Here's how the part is built. I have some questions about the finished solid (model axes, mm). Face numbers are marked on the shaded views. Round coordinates to 2 decimals unless told otherwise and drop trailing zeros. Loops run counter-clockwise (first coordinate to the right, second up) from the corner with the lowest first, then second, coordinate; pieces in that order, holes last. Notation, with made-up numbers: (-21, 0) - (21, 0) arc R16 ccw to (21, 16) - close; hole circle Ø10 at (31, 13). An arc over 180 degrees is marked (long way). Answer as a JSON object with one key per item and string values. Group by question number.
1) I want a section at C-C, the plane z = 1.55. Please give me the cut outline in (x, y).
2) I want a section at A-A, the plane y = 0. Please give me the cut outline in (x, z), then the cut area to 3 significant figures.
3) If I drill on line 1 along X through (y, z) = (0, 1.3); line 2 along Z through (x, y) = (5, 3); line 3 along X through (y, z) = (-8, 1.45), over which ranges is the centre line in solid material (lowest first)? Write a range as [from, to].
4) If we mould it in two halves opening along X, with no side actions, what happens to the marked faces 1 and 2? For each: pulls with the +X half, pulls with the -X half, needs draft (parallel to the pull), parting line crosses it, or undercut.
5) I want a section at B-B, the plane x = 0. Please give me the cut outline in (y, z), then the cut area to 3 significant figures.
6) Will these pins go through, and if not, where does the flat tip stop? P1, Ø8, axis at x = -4, y = 10, coming from the -Z side; P2, Ø1.5, axis at y = 15.5, z = 1.5, coming from the -X side; P3, Ø1.5, axis at x = -12, z = 1.5, coming from the +Y side; P4, Ø1, axis at x = -8, z = 2, coming from the +Y side.
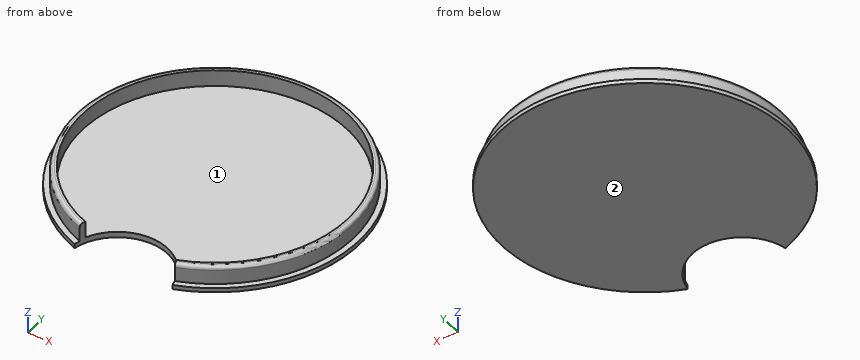
from build123d import *

# Parameters (mm, degrees)
F0_R     = 20
F1_DEPTH = 0.6
F3_R     = 19.2
F4_DEPTH = 2.5
F5_T     = -0.8
F6_R     = 0.5
F9_D     = 14
F9_DEPTH = 4


with BuildPart() as f1:
    # F0 (on Top) → F1 (new body)
    with BuildSketch(Plane.XY):
        Circle(F0_R)
    extrude(amount=F1_DEPTH)

    # F3 (on face) → F4 (join)
    with BuildSketch(Plane.XY.offset(0.6)):
        Circle(F3_R)
    extrude(amount=F4_DEPTH)

    # F5
    f5_openings = [f1.faces().sort_by_distance(p)[0] for p in [
        (0, 0, 3.1),
    ]]
    offset(amount=F5_T, openings=f5_openings)

    # F6
    f6_edges = [f1.edges().sort_by_distance(p)[0] for p in [
        (-19.2, 0, 3.1),
    ]]
    fillet(f6_edges, radius=F6_R)

    # F9
    with Locations(Plane.XY.offset(3.1)):
        with Locations((0, -20)):
            Hole(F9_D / 2, depth=F9_DEPTH)


solid = f1.part
Outcome:
{
 "1": {"outline": "(-6.71, -17.99) arc R7 cw to (-6.43, -17.24) arc R18.4 cw (long way) to (6.43, -17.24) arc R7 cw to (6.71, -17.99) arc R19.2 ccw (long way) to start"},
 "2": {"outline": "(-20, 0) - (20, 0) - (20, 0.6) - (19.2, 0.6) - (19.2, 2.6) arc R0.5 ccw to (18.7, 3.1) - (18.4, 3.1) - (18.4, 0.8) - (-18.4, 0.8) - (-18.4, 3.1) - (-18.7, 3.1) arc R0.5 ccw to (-19.2, 2.6) - (-19.2, 0.6) - (-20, 0.6) - close", "area": "35.3 mm^2"},
 "3": {"line 1": "[-19.2, -18.4], [18.4, 19.2]", "line 2": "[0, 0.8]", "line 3": "[-17.45, -16.57], [16.57, 17.45]"},
 "4": {"face 1": "undercut", "face 2": "needs draft"},
 "5": {"outline": "(-13, 0) - (20, 0) - (20, 0.6) - (19.2, 0.6) - (19.2, 2.6) arc R0.5 ccw to (18.7, 3.1) - (18.4, 3.1) - (18.4, 0.8) - (-13, 0.8) - close", "area": "28.0 mm^2"},
 "6": {"P1": "z = 0", "P2": "x = -12.29", "P3": "y = 15.56", "P4": "y = 17.67"}
}
